CAD build for the part. Positions are in the model's coordinates, mm. A direction names the side the tool comes from. Coordinates: 2 decimals unless noted, no trailing zeros. Loops run counter-clockwise (first coordinate to the right, second up) from the corner with the lowest first, then second, coordinate; pieces in that order, holes last.
1) Saw through at A-A, the plane z = 52.5. Write the cut outline in (x, y), and give its area (3 significant figures).
2) Which spindle directions (+Z, -Z, +X, -X, +Y, -Y) get a long thin tool onto all of the face, cutting with end or side? Do faces 1 (the cylindrical face through (-45.5, -2, -71.55)), 2 (the cylindrical face through (-11.436, -2.004, 68.436)), 3 (the cylindrical face through (-41.585, -2.004, 72.346)), 4 (the cylindrical face through (-56.53, -2, -70.31)). Say none if no direction does.
3) Two-plate mould, pull along X, no slides. Class faces 5 (the cylindrical face through (-58.94, -2, -72)), 6 (the cylindrical face through (-28.93, -2, 70.24)), 7 (the cylindrical face through (-6.128, -2.004, -33.211)): +X half, -X half, draft (parallel to the pull), parting line (faces both ways), or undercut.
4) Pin check, flat tips, straight feed: pin 1 Ø1.5 at (y, z) = (-1, -13.5) entering from -X; pin 2 Ø1.5 at (y, z) = (-2.5, -53.5) entering from -X. Stop position of each tip, or through.
5) Wall check: line 1 along X through (y, z) = (-1.2, -69); line 2 along Z through (x, y) = (-14, -2.5); line 3 along Z through (x, y) = (-40.5, -0.4). Give the ranges that are in metal, low to high.
6) Saw through at B-B, the plane z = 24. Write the cut outline in (x, y), and give its area (3 significant figures).
```python
from build123d import *

# Parameters (mm, degrees)
F1_DEPTH = 4.064


with BuildPart() as f1:
    # F0 (on Front) → F1 (new body)
    with BuildSketch(Plane.XZ):
        with BuildLine():
            ThreePointArc((-66.415959, 76.914086), (-67.172145, 76.691627), (-66.809714, 75.991663))
            ThreePointArc((-66.809714, 75.991663), (-66.017951, 74.646721), (-64.843036, 73.619425))
            ThreePointArc((-64.843036, 73.619425), (-64.666112, 69.398687), (-61.0939, 67.143641))
            ThreePointArc((-61.0939, 67.143641), (-66.055858, 56.303612), (-67.569681, 44.478402))
            ThreePointArc((-67.569681, 44.478402), (-70.50287, 40.806661), (-71.830064, 36.298465))
            ThreePointArc((-71.830064, 36.298465), (-70.238683, 36.587844), (-69.314263, 37.915128))
            ThreePointArc((-69.314263, 37.915128), (-69.520495, 36.197783), (-69.80937, 34.492392))
            ThreePointArc((-69.80937, 34.492392), (-68.738891, 34.449604), (-67.69567, 34.205791))
            ThreePointArc((-67.69567, 34.205791), (-68.644172, 31.540218), (-69.49908, 28.84317))
            ThreePointArc((-69.49908, 28.84317), (-72.946881, 22.816432), (-73.735699, 15.918123))
            ThreePointArc((-73.735699, 15.918123), (-75.910649, -4.322399), (-72.977036, -24.466952))
            ThreePointArc((-72.977036, -24.466952), (-70.518883, -42.867891), (-68.532197, -61.325684))
            ThreePointArc((-68.532197, -61.325684), (-66.688611, -64.841953), (-64.845026, -61.325684))
            ThreePointArc((-64.845026, -61.325684), (-62.852462, -60.158363), (-60.584038, -60.591031))
            ThreePointArc((-60.584038, -60.591031), (-62.366804, -64.333838), (-62.294377, -68.47891))
            ThreePointArc((-62.294377, -68.47891), (-60.351727, -68.232553), (-60.584038, -70.176932))
            ThreePointArc((-60.584038, -70.176932), (-58.918947, -72.027605), (-57.351563, -73.961727))
            ThreePointArc((-57.351563, -73.961727), (-56.146991, -74.041168), (-56.287132, -72.842141))
            ThreePointArc((-56.287132, -72.842141), (-56.528845, -70.272437), (-55.882256, -67.773692))
            ThreePointArc((-55.882256, -67.773692), (-54.520205, -64.167303), (-51.915128, -61.325684))
            ThreePointArc((-51.915128, -61.325684), (-50.51679, -63.617178), (-50.00503, -66.252401))
            ThreePointArc((-50.00503, -66.252401), (-48.412524, -69.353697), (-48.59242, -72.835328))
            ThreePointArc((-48.59242, -72.835328), (-47.924139, -73.806953), (-46.987015, -73.091094))
            ThreePointArc((-46.987015, -73.091094), (-45.486049, -71.528376), (-44.715524, -69.503214))
            ThreePointArc((-44.715524, -69.503214), (-43.721814, -65.468221), (-43.39315, -61.325684))
            ThreePointArc((-43.39315, -61.325684), (-44.513459, -58.166673), (-43.39315, -55.007663))
            ThreePointArc((-43.39315, -55.007663), (-35.936491, -56.266123), (-30.316319, -61.325684))
            ThreePointArc((-30.316319, -61.325684), (-29.359215, -64.47905), (-29.287802, -67.773692))
            ThreePointArc((-29.287802, -67.773692), (-27.447605, -71.320201), (-24.352325, -73.846719))
            ThreePointArc((-24.352325, -73.846719), (-23.889052, -75.343964), (-23.704438, -76.900333))
            ThreePointArc((-23.704438, -76.900333), (-23.092076, -77.454732), (-22.629103, -76.770626))
            ThreePointArc((-22.629103, -76.770626), (-22.69355, -70.344178), (-21.146461, -64.106397))
            ThreePointArc((-21.146461, -64.106397), (-16.406969, -67.834653), (-10.9533, -70.407622))
            ThreePointArc((-10.9533, -70.407622), (-9.080009, -73.063494), (-9.1583, -76.312609))
            ThreePointArc((-9.1583, -76.312609), (-6.332531, -71.75776), (-9.1583, -67.202911))
            ThreePointArc((-9.1583, -67.202911), (-11.807812, -61.726767), (-16.064042, -57.380209))
            ThreePointArc((-16.064042, -57.380209), (-12.202431, -49.388101), (-9.599092, -40.90232))
            ThreePointArc((-9.599092, -40.90232), (-6.08091, -33.101189), (-2.84028, -25.180737))
            ThreePointArc((-2.84028, -25.180737), (-0.994144, 2.976639), (-9.599092, 29.850435))
            ThreePointArc((-9.599092, 29.850435), (-10.261747, 31.2046), (-9.599092, 32.558765))
            ThreePointArc((-9.599092, 32.558765), (-8.917225, 34.568172), (-9.599092, 36.577579))
            ThreePointArc((-9.599092, 36.577579), (-8.189599, 36.500467), (-7.024208, 35.703924))
            ThreePointArc((-7.024208, 35.703924), (-8.593374, 45.18609), (-12.091408, 54.138046))
            ThreePointArc((-12.091408, 54.138046), (-13.067545, 56.145089), (-13.282336, 58.366559))
            ThreePointArc((-13.282336, 58.366559), (-12.146196, 58.89145), (-10.894712, 58.880817))
            ThreePointArc((-10.894712, 58.880817), (-12.661005, 60.885727), (-14.347583, 62.958144))
            ThreePointArc((-14.347583, 62.958144), (-13.617504, 63.466614), (-12.731345, 63.545868))
            ThreePointArc((-12.731345, 63.545868), (-13.158819, 65.019265), (-13.943524, 66.337548))
            ThreePointArc((-13.943524, 66.337548), (-11.402644, 68.467779), (-9.15432, 70.904784))
            ThreePointArc((-9.15432, 70.904784), (-9.381127, 71.904914), (-10.293034, 72.374091))
            ThreePointArc((-10.293034, 72.374091), (-9.485105, 73.019394), (-8.860459, 73.843397))
            ThreePointArc((-8.860459, 73.843397), (-8.522262, 74.402333), (-8.529865, 75.055577))
            ThreePointArc((-8.529865, 75.055577), (-14.055948, 74.882941), (-19.402735, 73.476076))
            ThreePointArc((-19.402735, 73.476076), (-22.695461, 72.250511), (-25.720755, 70.463993))
            ThreePointArc((-25.720755, 70.463993), (-28.977803, 70.239264), (-32.234851, 70.463993))
            ThreePointArc((-32.234851, 70.463993), (-34.548049, 70.692721), (-36.621001, 71.74442))
            ThreePointArc((-36.621001, 71.74442), (-41.655805, 72.345638), (-46.690609, 71.74442))
            ThreePointArc((-46.690609, 71.74442), (-47.679037, 71.017736), (-48.667464, 71.74442))
            ThreePointArc((-48.667464, 71.74442), (-51.942994, 74.141168), (-55.799965, 75.405002))
            ThreePointArc((-55.799965, 75.405002), (-61.025995, 76.736158), (-66.415959, 76.914086))
        make_face()
    extrude(amount=F1_DEPTH)


solid = f1.part
```
Data:
1. outline: (-66.94, -4.06) - (-11.29, -4.06) - (-11.29, 0) - (-66.94, 0) - close
1. area: 226 mm2
2. face 1: -Z, +Y, -Y
2. face 2: +X, +Y, -Y
2. face 3: +Z, +Y, -Y
2. face 4: +Y, -Y
3. face 5: -X half
3. face 6: undercut
3. face 7: +X half
4. pin 1: stops at x = -75.31
4. pin 2: stops at x = -69.4
5. line 1: x = -59.99 to -56.32, -48.5 to -44.55, -28.85 to -22.5, -14.32 to -7.15
5. line 2: z = -69.16 to -59.14, -53.5 to 62.52, 63.27 to 74.89
5. line 3: z = -54.98 to 72.31
6. outline: (-72.51, -4.06) - (-6.74, -4.06) - (-6.74, 0) - (-72.51, 0) - close
6. area: 267 mm2
